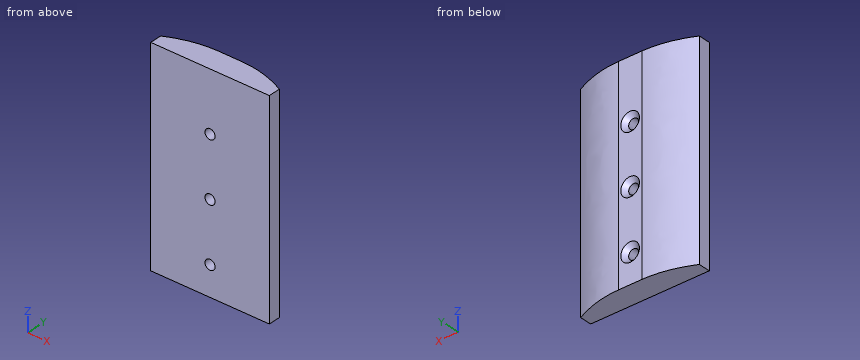
from build123d import *

# Parameters (mm, degrees)
SKETCH1_R                                       = 1.25
BOSS_EXTRUDE1_DEPTH                             = 4
BOSS_EXTRUDE2_DEPTH                             = 70
SKETCH3_R                                       = 1.6
SKETCH3_R_2                                     = 1.625
CUT_EXTRUDE1_DEPTH                              = 70
CSK_FOR_M3_FLAT_HEAD_MACHINE_SCREW1_D           = 3.4
CSK_FOR_M3_FLAT_HEAD_MACHINE_SCREW1_CSINK_D     = 6.3
CSK_FOR_M3_FLAT_HEAD_MACHINE_SCREW1_CSINK_ANGLE = 90


with BuildPart() as part:
    # Sketch1 → Boss-Extrude1 (new body)
    with BuildSketch(Plane(origin=(0, 0, 0), x_dir=(1, 0, 0), z_dir=(0, 1, 0))):
        Polygon((0, 35), (20, 35), (20, -35), (0, -35), (-20, -35), (-20, 35), align=None)
        with Locations(Location((0, 25, 0), (0, 0, 270))):
            Circle(SKETCH1_R, mode=Mode.SUBTRACT)
        with Locations(Location((0, 5, 0), (0, 0, 270))):
            Circle(SKETCH1_R, mode=Mode.SUBTRACT)
        with Locations(Location((0, -15, 0), (0, 0, 270))):
            Circle(SKETCH1_R, mode=Mode.SUBTRACT)
    extrude(amount=BOSS_EXTRUDE1_DEPTH)

    # Sketch2 → Boss-Extrude2 (add)
    with BuildSketch(Plane(origin=(0, 0, -35), x_dir=(-1, 0, 0), z_dir=(0, 0, -1))):
        with BuildLine():
            Line((0, 8), (-4, 8))
            add(Edge.make_bspline(
                [(-4, 8), (-9.652249971, 8), (-14.984519901, 6.51388548), (-20, 4)],
                knots=[0, 0, 0, 0, 1, 1, 1, 1], degree=3))
            Line((-20, 4), (20, 4))
            add(Edge.make_bspline(
                [(4, 8), (9.652249971, 8), (14.984519901, 6.51388548), (20, 4)],
                knots=[0, 0, 0, 0, 1, 1, 1, 1], degree=3))
            Line((4, 8), (0, 8))
        make_face()
    extrude(amount=-BOSS_EXTRUDE2_DEPTH)

    # Sketch3 → Cut-Extrude1 (cut)
    with BuildSketch(Plane(origin=(0, 8, 0), x_dir=(1, 0, 0), z_dir=(0, 1, 0))):
        with Locations(Location((0, 25, 0), (0, 0, 270))):
            Circle(SKETCH3_R)
        with Locations(Location((0, 5, 0), (0, 0, 270))):
            Circle(SKETCH3_R)
        with Locations(Location((0, -15, 0), (0, 0, 270))):
            Circle(SKETCH3_R_2)
    extrude(amount=-CUT_EXTRUDE1_DEPTH, mode=Mode.SUBTRACT)

    # CSK for M3 Flat Head Machine Screw1 (through all)
    with Locations(Plane(origin=(0, 8, 0), x_dir=(1, 0, 0), z_dir=(0, 1, 0))):
        with Locations((0, 25), (0, 5), (0, -15)):
            CounterSinkHole(CSK_FOR_M3_FLAT_HEAD_MACHINE_SCREW1_D / 2, CSK_FOR_M3_FLAT_HEAD_MACHINE_SCREW1_CSINK_D / 2, counter_sink_angle=CSK_FOR_M3_FLAT_HEAD_MACHINE_SCREW1_CSINK_ANGLE)


solid = part.part
Check sheet for the modelled part. Datum: model origin and axes. Units: mm. Round coordinates to 2 decimals unless told otherwise and drop trailing zeros. Write each loop counter-clockwise with the first axis right and the second up, starting at its lowest first coordinate (ties: lowest second). Pieces come first, ordered by that corner, then holes. Notation, with made-up numbers: (56.5, 13.25) - (107.5, 13.25) arc R14 ccw to (107.5, 27.25) - close; hole circle Ø11 at (82, 28.5). An arc over 180 degrees is marked (long way). Return JSON: item names as keys, results as strings.
Q1. Cross-section at B-B (y = 5.5). Give the number of separate pieces and of enclosed holes in the cut face, then the cut area to 3 significant figures.
Returned:
{"separate pieces": "1", "enclosed holes": "3", "area": "2,300 mm²"}
Q2. Scan lines: L1, parallel to Z at x = 0, y = 5; L2, parallel to Z at x = 1.5, y = 6.5; L3, parallel to X at y = 2, z = -5. Record each from-to range of solid material in increasing order. Write a range as from..to.
Returned:
{"L1": "z = -35..-26.7, -23.3..-6.7, -3.3..13.3, 16.7..35", "L2": "z = -35..-25.8, -24.2..-5.8, -4.2..14.2, 15.8..35", "L3": "x = -20..-1.7, 1.7..20"}
Q3. Cross-section at A-A (x = 0). Record the boundary of the cut face in (y, z), then the cut area to 3 significant figures.
Returned:
{"outline": "(0, -35) - (8, -35) - (8, -28.15) - (6.55, -26.7) - (0, -26.7) - close; (0, -23.3) - (6.55, -23.3) - (8, -21.85) - (8, -8.15) - (6.55, -6.7) - (0, -6.7) - close; (0, -3.3) - (6.55, -3.3) - (8, -1.85) - (8, 11.85) - (6.55, 13.3) - (0, 13.3) - close; (0, 16.7) - (6.55, 16.7) - (8, 18.15) - (8, 35) - (0, 35) - close", "area": "472 mm²"}
Q4. Depth check by flat-ended pin: P1, Ø4.5, axis at x = 0, z = 15, coming from the +Y side; P2, Ø2, axis at x = 1.5, z = -3.5, coming from the +Y side. Enter the tip coordinate at first touch or a pass-through.
Returned:
{"P1": "stops at y = 7.1", "P2": "stops at y = 7.97"}
